Read the model definition and answer for the solid it produces. Units are mm, in the model's axes. A direction names the side the tool comes from. Give positions to 0.01 mm unless a question says otherwise; leave off trailing zeros. Write each loop counter-clockwise with the first axis right and the second up, starting at its lowest first coordinate (ties: lowest second). Pieces come first, ordered by that corner, then holes.
```python
from build123d import *

# Parameters (mm, degrees)
BOSS_EXTRUDE6_DEPTH = 40
SKETCH9_R           = 16
CUT_EXTRUDE3_DEPTH  = 30
SKETCH10_R          = 16
CUT_EXTRUDE4_DEPTH  = 30
CUT_EXTRUDE5_REACH  = 89.959
SKETCH11_R          = 3.5
SKETCH12_R          = 11
CUT_EXTRUDE6_DEPTH  = 40
SKETCH14_W          = 106.764973624
SKETCH14_H          = 40
BOSS_EXTRUDE7_DEPTH = 5
CUT_EXTRUDE8_DEPTH  = 40
FILLET1_R           = 22
CHAMFER5_SIZE       = 2
CHAMFER6_SIZE       = 3
SKETCH16_R          = 5
CUT_EXTRUDE9_DEPTH  = 27


with BuildPart() as part:
    # Sketch8 → Boss-Extrude6 (new body)
    with BuildSketch(Plane.XY):
        Polygon((-57.969476198, -3.736595203), (37.23247397, 44.588846099), (50.811489539, 17.83795198), (-44.390460629, -30.487489322), align=None)
        Polygon((50.811489539, 17.83795198), (49.096562756, -22.125268937), (-11.118961612, -52.691258219), (-44.390460629, -30.487489322), align=None)
    extrude(amount=BOSS_EXTRUDE6_DEPTH)

    # Sketch9 → Cut-Extrude3 (cut)
    with BuildSketch(Plane(origin=(-27.75471112, -41.58937377, 0), x_dir=(-0.8317874754097543, 0.5550942224086534, 0), z_dir=(-0.5550942224086534, -0.8317874754097543, 0))):
        with Locations(Location((0, -20, 0), (0, 0, 180))):
            Circle(SKETCH9_R)
    extrude(amount=-CUT_EXTRUDE3_DEPTH, mode=Mode.SUBTRACT)

    # Sketch10 → Cut-Extrude4 (cut)
    with BuildSketch(Plane(origin=(49.954026147, -2.143658479, 0), x_dir=(0, 0, -1), z_dir=(0.9990805229464255, -0.04287316957138965, 0))):
        with Locations(Location((-20, 0, 0), (0, 0, 90))):
            Circle(SKETCH10_R)
    extrude(amount=-CUT_EXTRUDE4_DEPTH, mode=Mode.SUBTRACT)

    # Cut-Extrude5: up to this face of the body (flat: up to its plane)
    cut_extrude5_end = Plane(part.part.faces().sort_by_distance((3.278005206, -6.45772661, 40))[0])
    # Sketch11 → Cut-Extrude5 (cut, up to the picked face)
    with BuildSketch(Plane(origin=(0, 0, 0), x_dir=(-1, 0, 0), z_dir=(0, 0, -1)), mode=Mode.PRIVATE) as cut_extrude5_sk1:
        with Locations((16.072269088, -23.982451877)):
            Circle(SKETCH11_R)
    cut_extrude5_tool1 = split(extrude(cut_extrude5_sk1.sketch, amount=-CUT_EXTRUDE5_REACH, mode=Mode.PRIVATE), bisect_by=cut_extrude5_end, keep=Keep.BOTH, mode=Mode.PRIVATE)
    # Sketch11 → Cut-Extrude5 (cut, up to the picked face)
    with BuildSketch(Plane(origin=(0, 0, 0), x_dir=(-1, 0, 0), z_dir=(0, 0, -1)), mode=Mode.PRIVATE) as cut_extrude5_sk2:
        with Locations((22.894837472, -34.264871857)):
            Circle(SKETCH11_R)
    cut_extrude5_tool2 = split(extrude(cut_extrude5_sk2.sketch, amount=-CUT_EXTRUDE5_REACH, mode=Mode.PRIVATE), bisect_by=cut_extrude5_end, keep=Keep.BOTH, mode=Mode.PRIVATE)
    # Sketch11 → Cut-Extrude5 (cut, up to the picked face)
    with BuildSketch(Plane(origin=(0, 0, 0), x_dir=(-1, 0, 0), z_dir=(0, 0, -1)), mode=Mode.PRIVATE) as cut_extrude5_sk3:
        with Locations((-28.78289974, -1.065658383)):
            Circle(SKETCH11_R)
    cut_extrude5_tool3 = split(extrude(cut_extrude5_sk3.sketch, amount=-CUT_EXTRUDE5_REACH, mode=Mode.PRIVATE), bisect_by=cut_extrude5_end, keep=Keep.BOTH, mode=Mode.PRIVATE)
    # Sketch11 → Cut-Extrude5 (cut, up to the picked face)
    with BuildSketch(Plane(origin=(0, 0, 0), x_dir=(-1, 0, 0), z_dir=(0, 0, -1)), mode=Mode.PRIVATE) as cut_extrude5_sk4:
        with Locations((-41.131848905, -1.765246078)):
            Circle(SKETCH11_R)
    cut_extrude5_tool4 = split(extrude(cut_extrude5_sk4.sketch, amount=-CUT_EXTRUDE5_REACH, mode=Mode.PRIVATE), bisect_by=cut_extrude5_end, keep=Keep.BOTH, mode=Mode.PRIVATE)
    add(cut_extrude5_tool1.solids().sort_by(Axis((-16.072269, -23.982452, 0), (0, 0, 1)))[0], mode=Mode.SUBTRACT)
    add(cut_extrude5_tool2.solids().sort_by(Axis((-22.894837, -34.264872, 0), (0, 0, 1)))[0], mode=Mode.SUBTRACT)
    add(cut_extrude5_tool3.solids().sort_by(Axis((28.7829, -1.065658, 0), (0, 0, 1)))[0], mode=Mode.SUBTRACT)
    add(cut_extrude5_tool4.solids().sort_by(Axis((41.131849, -1.765246, 0), (0, 0, 1)))[0], mode=Mode.SUBTRACT)

    # Sketch12 → Cut-Extrude6 (cut)
    with BuildSketch(Plane(origin=(0, 0, 0), x_dir=(-1, 0, 0), z_dir=(0, 0, -1))):
        with Locations((0.002217481, -0.001125615)):
            Circle(SKETCH12_R)
    extrude(amount=-CUT_EXTRUDE6_DEPTH, mode=Mode.SUBTRACT)

    # Sketch14 → Boss-Extrude7 (add)
    with BuildSketch(Plane(origin=(-10.368501114, 20.426125448, 0), x_dir=(0.8916964706359383, 0.45263385230825515, 0), z_dir=(-0.45263385230825526, 0.8916964706359384, 0))):
        with Locations((0, -20)):
            Rectangle(SKETCH14_W, SKETCH14_H)
    extrude(amount=BOSS_EXTRUDE7_DEPTH)

    # Sketch15 → Cut-Extrude8 (cut)
    with BuildSketch(Plane(origin=(0, 0, 0), x_dir=(-1, 0, 0), z_dir=(0, 0, -1))):
        Polygon((20.486288281, 20.897526908), (10.387815393, 20.46417491), (44.390460629, -30.487489322), (60.232645459, 0.72188715), align=None)
        Polygon((-34.969304708, 49.047328453), (-50.811489539, 17.83795198), (10.387815393, 20.46417491), (4.777052471, 28.871688695), align=None)
        Polygon((4.777052471, 28.871688695), (10.387815393, 20.46417491), (20.486288281, 20.897526908), align=None)
    extrude(amount=-CUT_EXTRUDE8_DEPTH, mode=Mode.SUBTRACT)

    # Fillet1
    fillet1_edges = [part.edges().sort_by_distance(p)[0] for p in [
        (-10.387815393, 20.46417491, 20),
    ]]
    fillet(fillet1_edges, radius=FILLET1_R)

    # Chamfer5
    chamfer5_edges = [part.edges().sort_by_distance(p)[0] for p in [
        (49.096562756, -22.125268937, 20),
        (-11.118961612, -52.691258219, 20),
    ]]
    chamfer(chamfer5_edges, length=CHAMFER5_SIZE)

    # Chamfer6
    chamfer6_edges = [part.edges().sort_by_distance(p)[0] for p in [
        (50.811489539, 17.83795198, 20),
        (-44.390460629, -30.487489322, 20),
    ]]
    chamfer(chamfer6_edges, length=CHAMFER6_SIZE)

    # Sketch16 → Cut-Extrude9 (cut)
    with BuildSketch(Plane(origin=(18.988800572, -37.408263578, 0), x_dir=(-0.8916964706359382, -0.4526338523082556, 0), z_dir=(0.4526338523082556, -0.8916964706359382, 0))):
        with Locations(Location((-1.764586017, -20, 0), (0, 0, 180))):
            Circle(SKETCH16_R)
    extrude(amount=-CUT_EXTRUDE9_DEPTH, mode=Mode.SUBTRACT)


solid = part.part
```
Item 1: Find the intervals of material crossed by line 1 along X through (y, z) = (-22.5, 18); line 2 along Y through (x, z) = (-2.5, 10); line 3 along Y through (x, z) = (-4, 10), in increasing order.
Result set:
line 1: x = -39.06 to -34.1, -2.31 to 8.26, 18.54 to 47.65
line 2: y = -48.32 to -26.25, -22.38 to -10.71, 10.71 to 19.67
line 3: y = -49.08 to -28.49, -21.38 to -10.25, 10.25 to 19.37
Item 2: Determine the mould class of faces 3 (the cylindrical face through (-13.4, -33.39, 5.81)), 4 (the cylindrical face through (-8.78, 17.64, 20.28)), 5 (the cylindrical face through (13.57, -25.23, 15.12)), 6 (the flat face through (5, -11, 40)) for opening direction Z: pulls with the +Z half, pulls with the -Z half, needs draft (parallel to the pull), parting line crosses it, or undercut.
Result set:
face 3: undercut
face 4: needs draft
face 5: undercut
face 6: pulls with the +Z half
Item 3: Each of these flat-tipped pins is pushed along its axis until it touches: pin 1 Ø8 at (x, z) = (-32, 25) entering from +Y; pin 2 Ø6 at (y, z) = (-6.5, 28.5) entering from +X; pin 3 Ø5 at (x, y) = (32, -34) entering from +Z; pin 4 Ø2 at (x, z) = (-2, 24.5) entering from -Y. Where does it stop, or does it pass through?
Result set:
pin 1: stops at y = -5.93
pin 2: stops at x = 19.87
pin 3: passes through
pin 4: stops at y = -48.57
Item 4: Section B-B (z = 34.5) is taken. Write down the section's boundary in (x, y), and give its area (3 significant figures).
Result set:
outline: (-42.73, -27.99) - (-41.9, -32.15) - (-33.38, -37.83) - (-16.73, -12.88) - (-5.48, -20.39) - (-22.13, -45.34) - (-12.78, -51.58) - (-9.34, -51.79) - (47.31, -23.03) - (49.18, -20.13) - (49.66, -8.9) - (19.69, -7.62) - (20.27, 5.9) - (50.24, 4.61) - (50.68, 14.84) - (47.81, 17.97) - (1.98, 19.93) arc R22 ccw to (-17.26, 10.17) - close; hole circle Ø22 at (0, 0)
area: 3,410 mm2
Item 5: Which of the six approach directions +Z, -Z, +X, -X, +Y, -Y give full straight-line access (tool end or side, diameter ignored) to faces 1 (the flat face through (-11.29, -16.51, 20.22)), 2 (the cylindrical face through (-24.51, -37.37, 2.17))?
Result set:
face 1: none
face 2: +Z, -Z
Item 6: Section A-A (x = -4) is taken. Give the number of separate pieces and of enclosed holes in the cut face, and give its area (3 significant figures).
Result set:
separate pieces: 2
enclosed holes: 1
area: 1,660 mm2
